Model file for the job. Use its own axes, mm. Round coordinates to 2 decimals unless told otherwise and drop trailing zeros. Order: outer loops, then holes, each group sorted by start corner. A loop starts at its lowest first (then second) coordinate and runs counter-clockwise, first axis right, second up. Notation, with made-up numbers: (-31, 66.5) - (-27, 66.5) arc R19 cw to (-27, 81.5) - close; hole circle Ø6 at (1.5, 36). An arc over 180 degrees is marked (long way). Put each result on its own line as item: value. Start each with the question number.
Item 1: Saw through at C-C on z = -53. List the corners of the cut face in (x, y), plus the area to 3 significant figures.
Item 2: Probe probe 1 along X at (y, z) = (-0.85, -12.7) (3 decimals); probe 2 along Z at (x, y) = (21.59, -1.1); probe 3 along Z at (x, y) = (311, -4.5). List the from-to ranges inside material, lowest first.
Item 3: Saw through at A-A on y = -1.5. List the corners of the cut face in (x, z) (3 decimals), plus the area to 3 significant figures.
Item 4: Pin check, flat tip, straight feed: pin 1 Ø3 at (x, y) = (244.5, -1.5) entering from +Z. Stop position of the tip, or through.
```python
from build123d import *

# Parameters (mm, degrees)
F1_DEPTH       = 6.35
F3_D           = 6.35
F3_CSINK_D     = 13.208
F3_CSINK_ANGLE = 90
F4_SIZE        = 6.34999


# Not quite as in the source:
# - a fillet or chamfer is up to 0.001 mm smaller than in the source, because OpenCascade refuses the exact size


with BuildPart() as f1:
    # F0 (on Front) → F1 (new body)
    with BuildSketch(Plane.XZ):
        with BuildLine():
            Line((381, 0), (0, 0))
            Line((0, 0), (0, -58.9188076556))
            Line((0, -58.9188076556), (407.243362891, -19.705731858))
            ThreePointArc((407.243362891, -19.705731858), (411.7971966033, -15.2795473621), (408.473715423, -9.868171981))
            Line((408.473715423, -9.868171981), (381, 0))
        make_face()
    extrude(amount=F1_DEPTH)

    # F3 (through all)
    with Locations(Plane.XZ.offset(6.35)):
        with Locations((12.7, -12.7), (30.48, -12.7), (21.59, -28.0979316793)):
            CounterSinkHole(F3_D / 2, F3_CSINK_D / 2, counter_sink_angle=F3_CSINK_ANGLE)

    # F4 (size 6.35 in the source; OpenCascade refuses exactly that, so slightly less here)
    f4_edges = [f1.edges().sort_by_distance(p)[0] for p in [
        (190.5, 0, 0),
    ]]
    chamfer(f4_edges, length=F4_SIZE)


solid = f1.part
```
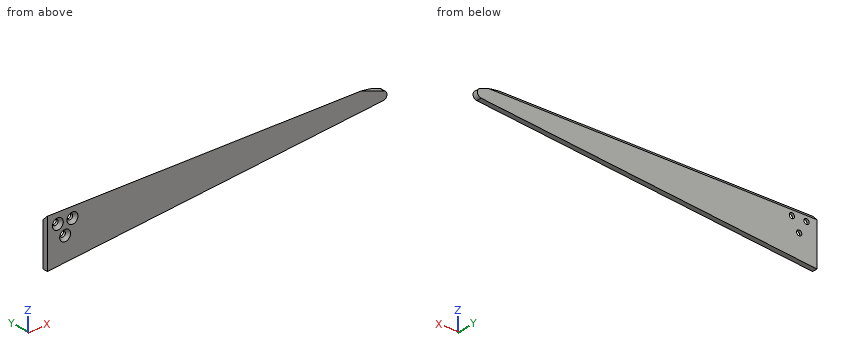
Results found:
1. outline: (0, -6.35) - (61.47, -6.35) - (61.47, 0) - (0, 0) - close
1. area: 390 mm²
2. probe 1: x = 0 to 9.525, 15.875 to 27.305, 33.655 to 411.448
2. probe 2: z = -56.84 to -31.27, -24.92 to -5.25
2. probe 3: z = -28.97 to -1.85
3. outline: (0, -58.919) - (407.243, -19.706) arc R5.08 ccw to (408.474, -9.868) - (394.503, -4.85) - (0, -4.85) - close; hole circle Ø6.35 at (12.7, -12.7); hole circle Ø6.35 at (21.59, -28.098); hole circle Ø6.35 at (30.48, -12.7)
3. area: 13,900 mm²
4. pin 1: stops at z = -3.35
